from build123d import *

# Parameters (mm, degrees)
SKETCH_R    = 6
PAD_DEPTH   = 3
FILLET_R    = 2
FILLET001_R = 1


with BuildPart() as part:
    # Sketch → Pad (new body)
    with BuildSketch(Plane.XY):
        Polygon((12.035368, 26.667595), (12.035368, -13.332405), (8.785368, -13.332405), (8.785368, -16.332405), (-1.114632, -16.332405), (-1.114632, -13.332405), (-41.214632, -13.332405), (-41.214632, -16.332405), (-51.114632, -16.332405), (-51.114632, -13.332405), (-54.364632, -13.332405), (-54.364632, 26.667595), (-51.114632, 26.667595), (-51.114632, 29.667595), (-41.214632, 29.667595), (-41.214632, 26.667595), (-1.114632, 26.667595), (-1.114632, 29.667595), (8.785368, 29.667595), (8.785368, 26.667595), align=None)
        with Locations((-45.167672, 14.667595)):
            Circle(SKETCH_R, mode=Mode.SUBTRACT)
        with Locations((-29.167672, 14.667595)):
            Circle(SKETCH_R, mode=Mode.SUBTRACT)
        with Locations((-13.167672, 14.667595)):
            Circle(SKETCH_R, mode=Mode.SUBTRACT)
        with Locations((2.832328, 14.667595)):
            Circle(SKETCH_R, mode=Mode.SUBTRACT)
    extrude(amount=PAD_DEPTH)

    # Fillet
    fillet_edges = [part.edges().sort_by_distance(p)[0] for p in [
        (-54.364632, 26.667595, 1.5),
        (-54.364632, -13.332405, 1.5),
        (12.035368, -13.332405, 1.5),
        (12.035368, 26.667595, 1.5),
    ]]
    fillet(fillet_edges, radius=FILLET_R)

    # Fillet001
    fillet001_edges = [part.edges().sort_by_distance(p)[0] for p in [
        (8.785368, 29.667595, 1.5),
        (-1.114632, 29.667595, 1.5),
        (-41.214632, 29.667595, 1.5),
        (-51.114632, 29.667595, 1.5),
        (-51.114632, -16.332405, 1.5),
        (-41.214632, -16.332405, 1.5),
        (-1.114632, -16.332405, 1.5),
        (8.785368, -16.332405, 1.5),
    ]]
    fillet(fillet001_edges, radius=FILLET001_R)


solid = part.part
Geometry check sheet. Reference: the model listing, model coordinates, mm. A direction names the side the tool comes from. Coordinates: 2 decimals unless noted, no trailing zeros. Loops run counter-clockwise (first coordinate to the right, second up) from the corner with the lowest first, then second, coordinate; pieces in that order, holes last. Notation, with made-up numbers: (89, 16) - (141, 16) arc R15 ccw to (141, 40) - close; hole circle Ø7 at (35, -13). An arc over 180 degrees is marked (long way). Use one line per item in the form item = value. Start each with the question number.
Item 1: Thickness scan on probe 1 along X at (y, z) = (13, 2.05); probe 2 along X at (y, z) = (17.5, 0.7); probe 3 along Y at (x, z) = (-0.5, 2.75). Record the ranges inside material, lowest first.
Item 2: Mould release check, pull along X, two halves, no side actions. Record for faces 1 (the face through (-41.215, -14, 1)), 2 (the face through (-51.115, -14, 1)), 3 (the face through (11.465, -12.731, 1.521)), 4 (the face through (-41.215, 28, 1)): +X half, -X half, draft (parallel to the pull), parting line (faces both ways), or undercut.
Item 3: Section check A-A, the plane x = -32. Enter the section's corners in (y, z), and give its area (3 significant figures).
Item 4: Section check D-D, the plane z = 0.7. Give the number of separate pieces and of enclosed holes in the cut face, and give its area (3 significant figures).
Item 5: Section check B-B, the plane y = 13. Enter the section's corners in (x, z).
Item 6: Section check C-C, the plane x = 6.5. Enter the section's corners in (y, z).
Item 7: Gauge pin test, flat ends, axial feed: pin 1 (1 mm diameter, centred on y = 27.5, z = 1, fed in from -X); pin 2 (0.9 mm diameter, centred on x = -26, z = 2, fed in from +Y); pin 3 (1 mm diameter, centred on x = -33, z = 1, fed in from -Y). Record the tip position at first contact, or that the pin passes through.
Item 8: Tool access check on faces 5 (the face through (8.785, -14, 1)), 6 (the face through (-52, -13.332, 1)), 7 (the face through (8.785, 28, 1)), 8 (the face through (-21, 26.668, 1)), 9 (the face through (-51.115, 28, 1)). Record the directions out of +Z, -Z, +X, -X, +Y, -Y that give a thin tool (end or side, any length) a straight path to the whole face; none if there is none.
Computed:
q1.probe_1 = -54.36 to -50.93, -39.4 to -34.93, -23.4 to -18.93, -7.4 to -2.93, 8.6 to 12.04
q1.probe_2 = -54.36 to -50.46, -39.88 to -34.46, -23.88 to -18.46, -7.88 to -2.46, 8.12 to 12.04
q1.probe_3 = -16.26 to 9.68, 19.66 to 29.59
q2.face_1 = undercut
q2.face_2 = -X half
q2.face_3 = +X half
q2.face_4 = undercut
q3.outline = (-13.33, 0) - (9.38, 0) - (9.38, 3) - (-13.33, 3) - close; (19.96, 0) - (26.67, 0) - (26.67, 3) - (19.96, 3) - close
q3.area = 88.3 mm2
q4.separate_pieces = 1
q4.enclosed_holes = 4
q4.area = 2,320 mm2
q5.outline = (-54.36, 0) - (-50.93, 0) - (-50.93, 3) - (-54.36, 3) - close; (-39.4, 0) - (-34.93, 0) - (-34.93, 3) - (-39.4, 3) - close; (-23.4, 0) - (-18.93, 0) - (-18.93, 3) - (-23.4, 3) - close; (-7.4, 0) - (-2.93, 0) - (-2.93, 3) - (-7.4, 3) - close; (8.6, 0) - (12.04, 0) - (12.04, 3) - (8.6, 3) - close
q6.outline = (-16.33, 0) - (9.92, 0) - (9.92, 3) - (-16.33, 3) - close; (19.42, 0) - (29.67, 0) - (29.67, 3) - (19.42, 3) - close
q7.pin_1 = -51.11
q7.pin_2 = 26.67
q7.pin_3 = -13.33
q8.face_5 = +Z, -Z, +X, -Y
q8.face_6 = +Z, -Z, -X, -Y
q8.face_7 = +Z, -Z, +X, +Y
q8.face_8 = +Z, -Z, +Y
q8.face_9 = +Z, -Z, -X, +Y
